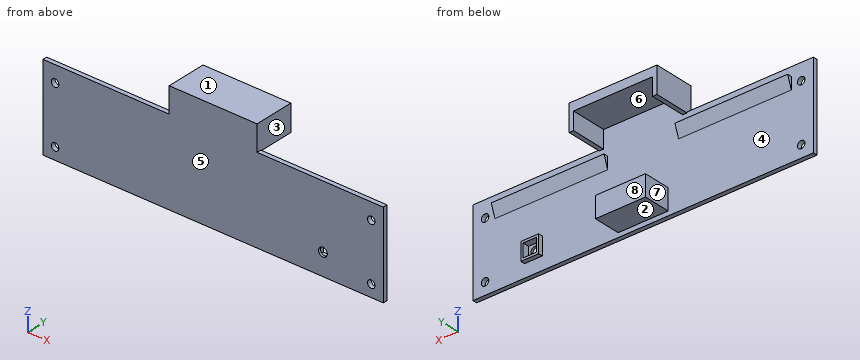
```python
from build123d import *

# Parameters (mm, degrees)
SKETCH043_W     = 155
SKETCH043_H     = 39
PAD008_DEPTH    = 2
SKETCH044_W     = 22.8
SKETCH044_H     = 9.5
PAD009_DEPTH    = 12.3
PAD011_DEPTH    = 51.35
SKETCH052_W     = 6.1
SKETCH052_H     = 6.1
POCKET011_DEPTH = 1
SKETCH053_R     = 2
POCKET012_DEPTH = 2.001
SKETCH065_W     = 40
SKETCH065_H     = 12
PAD020_DEPTH    = 2
PAD021_DEPTH    = 16.3
SKETCH069_R     = 1.7
POCKET016_DEPTH = 2
SKETCH079_W     = 8.1
SKETCH079_H     = 8.1
SKETCH079_W_2   = 6.1
SKETCH079_H_2   = 6.1
PAD025_DEPTH    = 2


with BuildPart() as part:
    # Sketch043 → Pad008 (new body)
    with BuildSketch(Plane.XZ):
        with Locations((0, -15.5)):
            Rectangle(SKETCH043_W, SKETCH043_H)
    extrude(amount=PAD008_DEPTH)

    # Sketch044 → Pad009 (join)
    with BuildSketch(Plane.XZ):
        with Locations((0, -28.25)):
            Rectangle(SKETCH044_W, SKETCH044_H)
    extrude(amount=-PAD009_DEPTH)

    # Sketch046 (on DatumPlane) → Pad011 (join)
    with BuildSketch(Plane.YZ.offset(-16.15)):
        Polygon((0, 0), (2, 0), (0, -5.494955), align=None)
    pad011 = extrude(amount=-PAD011_DEPTH)

    # Mirrored005: Pad011 across YZ
    add(pad011.mirror(Plane.YZ))

    # Sketch052 → Pocket011 (cut)
    with BuildSketch(Plane.XZ):
        with Locations((50, -25)):
            Rectangle(SKETCH052_W, SKETCH052_H)
    extrude(amount=POCKET011_DEPTH, mode=Mode.SUBTRACT)

    # Sketch053 → Pocket012 (cut, through all)
    with BuildSketch(Plane.XZ):
        with Locations((50, -25)):
            Circle(SKETCH053_R)
    extrude(amount=POCKET012_DEPTH, mode=Mode.SUBTRACT)

    # Sketch065 → Pad020 (join)
    with BuildSketch(Plane.XZ):
        with Locations((0, 9.6)):
            Rectangle(SKETCH065_W, SKETCH065_H)
    extrude(amount=PAD020_DEPTH)

    # Sketch066 → Pad021 (join)
    with BuildSketch(Plane.XZ):
        Polygon((-20, 3.6), (-20, 15.6), (20, 15.6), (20, 3.6), (18, 3.6), (18, 11.6), (-18, 11.6), (-18, 3.6), align=None)
    extrude(amount=-PAD021_DEPTH)

    # Sketch069 → Pocket016 (cut)
    with BuildSketch(Plane.XZ):
        with Locations((-72, -3.5)):
            Circle(SKETCH069_R)
        with Locations((-72, -29.5)):
            Circle(SKETCH069_R)
    pocket016 = extrude(amount=POCKET016_DEPTH, mode=Mode.SUBTRACT)

    # Mirrored010: Pocket016 across Sketch069 V_Axis
    add(pocket016.mirror(Plane(origin=(0, 0, 0), x_dir=(0, -1, 0), z_dir=(1, 0, 0))), mode=Mode.SUBTRACT)

    # Sketch079 → Pad025 (join)
    with BuildSketch(Plane.XZ):
        with Locations((50, -25)):
            Rectangle(SKETCH079_W, SKETCH079_H)
        with Locations((50, -25)):
            Rectangle(SKETCH079_W_2, SKETCH079_H_2, mode=Mode.SUBTRACT)
    extrude(amount=-PAD025_DEPTH)


with BuildPart() as part_1:
    # Body005 placement: moved
    add(part.part.moved(Location((0, -140, 0))))


solid = part_1.part
```
Verification items for the finished model (mm, model axes). Face numbers are marked on the shaded views. A direction names the side the tool comes from. Coordinates: 2 decimals unless noted, no trailing zeros. Order: outer loops, then holes, each group sorted by start corner. A loop starts at its lowest first (then second) coordinate and runs counter-clockwise, first axis right, second up. Notation, with made-up numbers: (32, 35) -> (78, 35) arc R20 cw to (78, 60) -> close; hole circle Ø7 at (60, 12). An arc over 180 degrees is marked (long way). Put each result on its own line as item: value. Start each with the question number.
1) Cross-section at D-D (x = -72). Enter the section's corners in (y, z).
2) Release check for a two-part mould opening along Z. For the marked faces 1, 2, 3 and 4 record: pulls with the +Z half, pulls with the -Z half, needs draft (parallel to the pull), parting line crosses it, or undercut.
3) Cross-section at C-C (x = 50). Enter the section's corners in (y, z), plus the area to 3 significant figures.
4) Cross-section at B-B (z = -25). Enter the section's corners in (x, y).
5) Material ranges on L1, parallel to Z at x = -72, y = -141.6; L2, parallel to Z at x = 50, y = -141.35; L3, parallel to X at y = -141.7, z = -25, recorded low to high.
6) Go/stop test with flat-tipped pins: pin 1 (4 mm diameter, centred on x = -72, z = -29.5, fed in from +Y); pin 2 (0.9 mm diameter, centred on y = -139.5, z = -26.5, fed in from +X); pin 3 (2 mm diameter, centred on x = -39, y = -138.5, fed in from +Z); pin 4 (3.5 mm diameter, centred on x = 49, y = -139, fed in from -Z). Record where each tip stops, or that it passes through.
7) Cross-section at A-A (y = -129.25). Enter the section's corners in (x, z), plus the area to 3 significant figures.
8) Tool access check on the marked faces 5, 6, 7 and 8. Record the directions out of +Z, -Z, +X, -X, +Y, -Y that give a thin tool (end or side, any length) a straight path to the whole face; none if there is none.
Geometry check:
1. outline: (-142, -35) -> (-140, -35) -> (-140, -31.2) -> (-142, -31.2) -> close; (-142, -27.8) -> (-140, -27.8) -> (-140, -5.2) -> (-142, -5.2) -> close; (-142, -1.8) -> (-140, -1.8) -> (-140, 4) -> (-142, 4) -> close
2. face 1: pulls with the +Z half
2. face 2: pulls with the -Z half
2. face 3: needs draft
2. face 4: undercut
3. outline: (-142, -35) -> (-140, -35) -> (-140, -29.05) -> (-138, -29.05) -> (-138, -28.05) -> (-141, -28.05) -> (-141, -27) -> (-142, -27) -> close; (-142, -23) -> (-141, -23) -> (-141, -21.95) -> (-138, -21.95) -> (-138, -20.95) -> (-140, -20.95) -> (-140, -5.49) -> (-138, 0) -> (-140, 0) -> (-140, 4) -> (-142, 4) -> close
3. area: 77.4 mm^2
4. outline: (-77.5, -142) -> (48, -142) -> (48, -141) -> (46.95, -141) -> (46.95, -138) -> (45.95, -138) -> (45.95, -140) -> (11.4, -140) -> (11.4, -127.7) -> (-11.4, -127.7) -> (-11.4, -140) -> (-77.5, -140) -> close; (52, -142) -> (77.5, -142) -> (77.5, -140) -> (54.05, -140) -> (54.05, -138) -> (53.05, -138) -> (53.05, -141) -> (52, -141) -> close
5. L1: z = -35 to -31.2, -27.8 to -5.2, -1.8 to 4
5. L2: z = -35 to -27, -23 to 4
5. L3: x = -77.5 to 48, 52 to 77.5
6. pin 1: stops at y = -140
6. pin 2: stops at x = 54.05
6. pin 3: stops at z = 0
6. pin 4: stops at z = -35
7. outline: (-20, 3.6) -> (-18, 3.6) -> (-18, 11.6) -> (18, 11.6) -> (18, 3.6) -> (20, 3.6) -> (20, 15.6) -> (-20, 15.6) -> close; (-11.4, -33) -> (11.4, -33) -> (11.4, -23.5) -> (-11.4, -23.5) -> close
7. area: 409 mm^2
8. face 5: +Z, -Z, +X, -X, -Y
8. face 6: +Y
8. face 7: -Z, -X, +Y
8. face 8: -Z, +X, -X, +Y
